The model under review builds one solid part; all positions refer to its coordinate system, in mm. Round coordinates to 2 decimals unless told otherwise and drop trailing zeros. Write each loop counter-clockwise with the first axis right and the second up, starting at its lowest first coordinate (ties: lowest second). Pieces come first, ordered by that corner, then holes. Notation, with made-up numbers: (6, 87) - (65, 87) arc R23 ccw to (65, 126) - close; hole circle Ø1 at (-24.5, 39). An arc over 180 degrees is marked (long way). Return JSON: item names as keys, results as strings.
from build123d import *

# Parameters (mm, degrees)
SKETCH1_W               = 45
SKETCH1_H               = 60
BOSS_EXTRUDE1_DEPTH     = 2.5
CUT_EXTRUDE1_DEPTH      = 38.831864876
CUT_EXTRUDE1_DEPTH_BACK = 38.831864876
SKETCH2_W               = 8.5
SKETCH2_H               = 5.5
CUT_EXTRUDE2_DEPTH      = 48.312788969
CUT_EXTRUDE2_DEPTH_BACK = 48.312788969
SKETCH9_R               = 1
FILLET1_R               = 2.5
CUT_EXTRUDE3_DEPTH      = 38.831864876
CUT_EXTRUDE3_DEPTH_BACK = 38.831864876
SKETCH13_W              = 15
SKETCH13_H              = 3
CUT_EXTRUDE4_START      = -6
SKETCH11_R              = 1.5
CUT_EXTRUDE4_DEPTH      = 59.08166664


with BuildPart() as part:
    # Sketch1 → Boss-Extrude1 (new, symmetric)
    with BuildSketch(Plane(origin=(0, 0, 0), x_dir=(1, 0, 0), z_dir=(0, 1, 0))):
        Rectangle(SKETCH1_W, SKETCH1_H)
    extrude(amount=BOSS_EXTRUDE1_DEPTH, both=True)

    # Sketch2 → Cut-Extrude1 (cut, two sides: drawn at the far end of the back side and taken through both)
    with BuildSketch(Plane(origin=(0, 2.5, 0), x_dir=(1, 0, 0), z_dir=(0, 1, 0)).offset(-CUT_EXTRUDE1_DEPTH_BACK)):
        with Locations((-18.25, -27.25)):
            Rectangle(SKETCH2_W, SKETCH2_H)
        with Locations((18.25, -27.25)):
            Rectangle(SKETCH2_W, SKETCH2_H)
    extrude(amount=CUT_EXTRUDE1_DEPTH + CUT_EXTRUDE1_DEPTH_BACK, mode=Mode.SUBTRACT)

    # Sketch9 → Cut-Extrude2 (cut, two sides: drawn at the far end of the back side and taken through both)
    with BuildSketch(Plane.ZY.offset(14).offset(-CUT_EXTRUDE2_DEPTH_BACK)):
        with Locations(Location((27, 0, 0), (0, 0, 180))):
            Circle(SKETCH9_R)
    extrude(amount=CUT_EXTRUDE2_DEPTH + CUT_EXTRUDE2_DEPTH_BACK, mode=Mode.SUBTRACT)

    # Fillet1
    fillet1_edges = [part.edges().sort_by_distance(p)[0] for p in [
        (-22.5, 2.5, -2.75),
        (22.5, -2.5, -2.75),
        (0, -2.5, 30),
        (22.5, 2.5, -2.75),
        (0, 2.5, 30),
        (-18.25, 2.5, 24.5),
        (-18.25, -2.5, 24.5),
        (-22.5, 0, 24.5),
        (18.25, 2.5, 24.5),
        (22.5, 0, 24.5),
        (18.25, -2.5, 24.5),
        (-22.5, -2.5, -2.75),
        (0, -2.5, -30),
        (0, 2.5, -30),
    ]]
    fillet(fillet1_edges, radius=FILLET1_R - 0.0001)  # a hair under: the kernel refuses the full size

    # Sketch13 → Cut-Extrude3 (cut, two sides: drawn at the far end of the back side and taken through both)
    with BuildSketch(Plane.XZ.offset(2.5).offset(-CUT_EXTRUDE3_DEPTH_BACK)):
        with Locations((0, 17.5)):
            Rectangle(SKETCH13_W, SKETCH13_H)
    extrude(amount=CUT_EXTRUDE3_DEPTH + CUT_EXTRUDE3_DEPTH_BACK, mode=Mode.SUBTRACT)

    # Sketch11 → Cut-Extrude4 (cut)
    with BuildSketch(Plane(origin=(20, 0, 0), x_dir=(0, 0, -1), z_dir=(1, 0, 0)).offset(CUT_EXTRUDE4_START)):
        with Locations((-5, 0)):
            Circle(SKETCH11_R)
    cut_extrude4 = extrude(amount=CUT_EXTRUDE4_DEPTH, mode=Mode.SUBTRACT)

    # Mirror1: Cut-Extrude4 across plane
    add(cut_extrude4.mirror(Plane(origin=(0, 0, 0), x_dir=(0, 0, 1), z_dir=(1, 0, 0))), mode=Mode.SUBTRACT)


solid = part.part
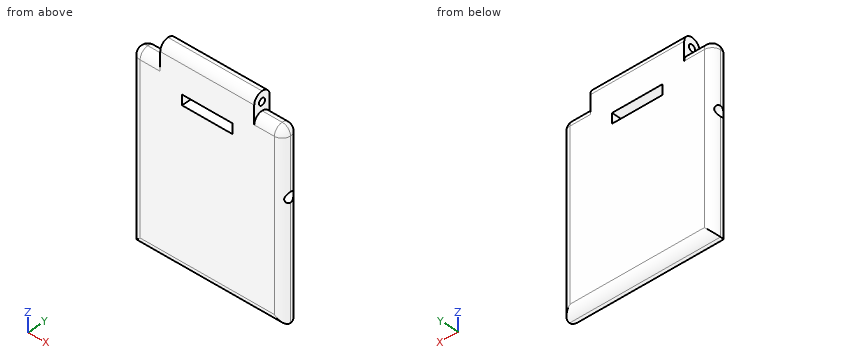
(1) Wall thickness on line 1 (Z direction, x = 19.25, y = 0); line 2 (Y direction, x = 7, z = 27); line 3 (Z direction, x = -9, y = -0.75): over which ranges is each line inside the solid? List them lowest first.
Filled in:
{"line 1": "z = -30 to 3.5, 6.5 to 24.5", "line 2": "y = -2.5 to -1, 1 to 2.5", "line 3": "z = -29.88 to 26.34, 27.66 to 29.88"}
(2) Add section D-D (z = 5). Write out the cut boundary in (x, y), plus the area to 3 significant figures.
Filled in:
{"outline": "(-22, -1.5) arc R2.5 ccw to (-20, -2.5) - (20, -2.5) arc R2.5 ccw to (22, -1.5) - (14, -1.5) - (14, 1.5) - (22, 1.5) arc R2.5 ccw to (20, 2.5) - (-20, 2.5) arc R2.5 ccw to (-22, 1.5) - (-14, 1.5) - (-14, -1.5) - close", "area": "170 mm2"}
(3) Clearance check with flat-ended pins moving along their axes: pin 1 Ø2.5 at (y, z) = (0, 5) entering from +X; pin 2 Ø2.5 at (y, z) = (0, 27) entering from -X; pin 3 Ø1.5 at (x, y) = (-16.5, -1.5) entering from -Z; pin 4 Ø1.5 at (y, z) = (0, 27) entering from -X. State where each tip first meets the part, or that it passes through.
Filled in:
{"pin 1": "stops at x = 14", "pin 2": "stops at x = -14", "pin 3": "stops at z = -29.88", "pin 4": "passes through"}
(4) Add section B-B (x = -2.5). Give the number of separate pieces and of enclosed holes in the cut face, plus the area to 3 significant figures.
Filled in:
{"separate pieces": "2", "enclosed holes": "1", "area": "276 mm2"}
